```python
from build123d import *

# Parameters (mm, degrees)
SKETCH_1_R               = 142.5
SKETCH_1_R_2             = 80
EXTRUDE_1_DEPTH          = 160
CUT_EXTRUDE_START        = -10
CUT_EXTRUDE_1_DEPTH      = 10
PATTERN_CIRCULAR_1_COUNT = 4
CUT_EXTRUDE_2_DEPTH      = 258.317896774
CUT_EXTRUDE_2_DEPTH_BACK = 258.317896774
SKETCH_3_W               = 17.844530797
SKETCH_3_H               = 166.856843943
SKETCH_3_W_2             = 22.841371227
CUT_EXTRUDE_3_REACH      = 346.683
CUT_EXTRUDE_3_END_RADIUS = 80
SKETCH_4_R               = 8.5


with BuildPart() as part:
    # 草图1 → 凸台-拉伸1 (new body)
    with BuildSketch(Plane(origin=(0, 0, 0), x_dir=(1, 0, 0), z_dir=(0, 1, 0))):
        with Locations(Location((0, 0, 0), (0, 0, 270))):
            Circle(SKETCH_1_R)
        with Locations(Location((0, 0, 0), (0, 0, 270))):
            Circle(SKETCH_1_R_2, mode=Mode.SUBTRACT)
    extrude(amount=EXTRUDE_1_DEPTH)

    # 草图2 → 切除-拉伸1 (cut)
    with BuildSketch(Plane(origin=(0, 160, 0), x_dir=(1, 0, 0), z_dir=(0, 1, 0)).offset(CUT_EXTRUDE_START)):
        with BuildLine():
            Line((-54.532389112, 131.652833383), (-30.614674589, 73.910362601))
            ThreePointArc((-30.614674589, 73.910362601), (0, 80), (30.614674589, 73.910362601))
            Line((30.614674589, 73.910362601), (54.532389112, 131.652833383))
            ThreePointArc((54.532389112, 131.652833383), (0, 142.5), (-54.532389112, 131.652833383))
        make_face()
    cut_extrude_1 = extrude(amount=CUT_EXTRUDE_1_DEPTH, mode=Mode.SUBTRACT)

    # 阵列(圆周)1: 切除-拉伸1 ×4 about axis
    pattern_circular_1_axis = Axis((0, 160, 0), (0, -1, 0))
    for i in range(1, PATTERN_CIRCULAR_1_COUNT):
        add(cut_extrude_1.rotate(pattern_circular_1_axis, i * 360 / PATTERN_CIRCULAR_1_COUNT), mode=Mode.SUBTRACT)

    # 草图3 → 切除-拉伸2 (cut, two sides: drawn at the far end of the back side and taken through both)
    with BuildSketch(Plane(origin=(0, 0, 0), x_dir=(0, 0, -1), z_dir=(1, 0, 0)).offset(-CUT_EXTRUDE_2_DEPTH_BACK)):
        with Locations((143.922265399, 83.428421972)):
            Rectangle(SKETCH_3_W, SKETCH_3_H)
        with Locations((-146.420685613, 83.428421972)):
            Rectangle(SKETCH_3_W_2, SKETCH_3_H)
    extrude(amount=CUT_EXTRUDE_2_DEPTH + CUT_EXTRUDE_2_DEPTH_BACK, mode=Mode.SUBTRACT)

    # 切除-拉伸3: up to this cylinder (the profile starts outside it)
    cut_extrude_3_end = Plane(origin=(0, 57.5, 0), z_dir=(0, -1, 0)) * Cylinder(CUT_EXTRUDE_3_END_RADIUS, 919.366, mode=Mode.PRIVATE)
    # 草图4 → 切除-拉伸3 (cut, up to the surface)
    with BuildSketch(Plane.XY.offset(135), mode=Mode.PRIVATE) as cut_extrude_3_sk1:
        with Locations((-30, 90)):
            Circle(SKETCH_4_R)
    cut_extrude_3_tool1 = extrude(cut_extrude_3_sk1.sketch, amount=-CUT_EXTRUDE_3_REACH, mode=Mode.PRIVATE) - cut_extrude_3_end
    # 草图4 → 切除-拉伸3 (cut, up to the surface)
    with BuildSketch(Plane.XY.offset(135), mode=Mode.PRIVATE) as cut_extrude_3_sk2:
        with Locations((30, 90)):
            Circle(SKETCH_4_R)
    cut_extrude_3_tool2 = extrude(cut_extrude_3_sk2.sketch, amount=-CUT_EXTRUDE_3_REACH, mode=Mode.PRIVATE) - cut_extrude_3_end
    # 草图4 → 切除-拉伸3 (cut, up to the surface)
    with BuildSketch(Plane.XY.offset(135), mode=Mode.PRIVATE) as cut_extrude_3_sk3:
        with Locations((30, 25)):
            Circle(SKETCH_4_R)
    cut_extrude_3_tool3 = extrude(cut_extrude_3_sk3.sketch, amount=-CUT_EXTRUDE_3_REACH, mode=Mode.PRIVATE) - cut_extrude_3_end
    # 草图4 → 切除-拉伸3 (cut, up to the surface)
    with BuildSketch(Plane.XY.offset(135), mode=Mode.PRIVATE) as cut_extrude_3_sk4:
        with Locations((-30, 25)):
            Circle(SKETCH_4_R)
    cut_extrude_3_tool4 = extrude(cut_extrude_3_sk4.sketch, amount=-CUT_EXTRUDE_3_REACH, mode=Mode.PRIVATE) - cut_extrude_3_end
    cut_extrude_3 = cut_extrude_3_tool1.solids().sort_by_distance((-30, 90, 135))[0] + cut_extrude_3_tool2.solids().sort_by_distance((30, 90, 135))[0] + cut_extrude_3_tool3.solids().sort_by_distance((30, 25, 135))[0] + cut_extrude_3_tool4.solids().sort_by_distance((-30, 25, 135))[0]
    add(cut_extrude_3, mode=Mode.SUBTRACT)

    # 镜向1: 切除-拉伸3 across plane
    add(cut_extrude_3.mirror(Plane.XY), mode=Mode.SUBTRACT)


solid = part.part
```
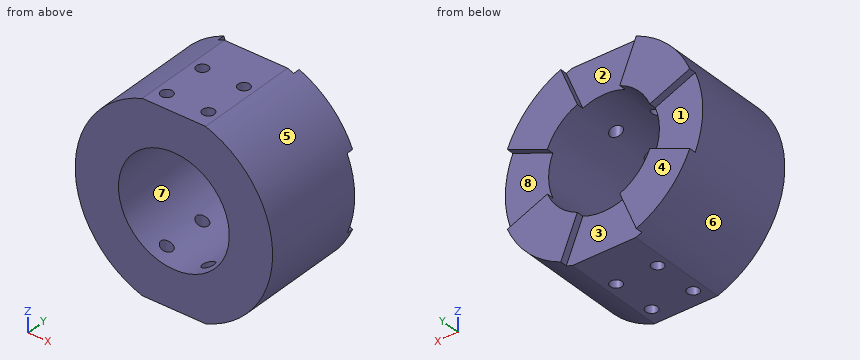
Geometry check sheet. Reference: the model listing, model coordinates, mm. Face numbers are marked on the shaded views. A direction names the side the tool comes from. Coordinates: 2 decimals unless noted, no trailing zeros. Write each loop counter-clockwise with the first axis right and the second up, starting at its lowest first coordinate (ties: lowest second). Pieces come first, ordered by that corner, then holes. Notation, with made-up numbers: M -7,85 L 3,85 A12 cw 3,106 Z; hole C 31,16.25 d5. An arc over 180 degrees is marked long. Use one line per item in the form item = value. Start each with the question number.
1) Section check B-B on y = 111. Enter the section's corners in (x, z), and give its area (3 significant figures).
2) Section check A-A on x = -63. Enter the section's corners in (y, z).
3) Go/stop test with flat-tipped pins: pin 1 Ø20.5 at (x, z) = (-100.5, 21.5) entering from +Y; pin 2 Ø10 at (y, z) = (32.5, -26) entering from +X; pin 3 Ø13.5 at (x, y) = (-30, 90) entering from +Z; pin 4 Ø4 at (x, y) = (-77.5, 142.5) entering from +Z. Record where each tip stops, or that it passes through.
4) Release check for a two-part mould opening along X. For the marked faces 5, 6, 7 and 8 record: pulls with the +X half, pulls with the -X half, needs draft (parallel to the pull), parting line crosses it, or undercut.
5) Thickness scan on probe 1 along Y at (x, z) = (30, -106); probe 2 along Z at (x, y) = (-2, 92) (3 decimals); probe 3 along Y at (x, z) = (36.5, 87). Record the ranges inside material, lowest first. Write a range as from..to.
6) Set-up check for the marked faces 1, 2, 3 and 4: record each of +Z, -Z, +X, -X, +Y, -Y from which the full face is reachable in a straight line by a thin tool's end or side.
7) Section check C-C on z = -43.5. Enter the section's corners in (x, y).
8) Section check D-D on y = 25. Enter the section's corners in (x, z).
Responses:
q1.outline = M -45.62,-135 L 45.62,-135 A142.5 ccw 45.62,135 L -45.62,135 A142.5 ccw Z; hole C 0,0 d160
q1.area = 42,800 mm2
q2.outline = M 0,-127.82 L 160,-127.82 L 160,-49.31 L 0,-49.31 Z; M 0,49.31 L 160,49.31 L 160,127.82 L 0,127.82 Z
q3.pin_1 = 150
q3.pin_2 = 140.94
q3.pin_3 = through
q3.pin_4 = 120.86
q4.face_5 = pulls with the +X half
q4.face_6 = pulls with the -X half
q4.face_7 = undercut
q4.face_8 = needs draft
q5.probe_1 = 0..16.5, 33.5..81.5, 98.5..150
q5.probe_2 = -135..-79.975, 79.975..135
q5.probe_3 = 0..19.52, 30.48..84.52, 95.48..160
q6.face_1 = -X, +Y
q6.face_2 = +Z, +Y
q6.face_3 = -Z, +Y
q6.face_4 = +Z, -Z, +X, -X, +Y
q7.outline = M -135.7,0 L -67.14,0 L -67.14,160 L -105.02,160 L -105.02,150 L -135.7,150 Z; M 67.14,0 L 135.7,0 L 135.7,150 L 105.02,150 L 105.02,160 L 67.14,160 Z
q8.outline = M -45.62,-135 L -38.5,-135 L -38.5,-70.13 A80 cw -38.5,70.13 L -38.5,135 L -45.62,135 A142.5 ccw Z; M -21.5,-135 L 21.5,-135 L 21.5,-77.06 A80 cw -21.5,-77.06 Z; M -21.5,77.06 A80 cw 21.5,77.06 L 21.5,135 L -21.5,135 Z; M 38.5,-135 L 45.62,-135 A142.5 ccw 45.62,135 L 38.5,135 L 38.5,70.13 A80 cw 38.5,-70.13 Z
